Drawing for the job (mm, zero at the part's lowest x, y, z). A direction names the side the tool comes from. Give positions to 0.01 mm unless a question says otherwise; leave off trailing zeros. Write each loop counter-clockwise with the first axis right and the second up, starting at its lowest first coordinate (ties: lowest second). Pieces come first, ordered by that corner, then holes. Notation, with made-up numbers: (-6, 42.25) - (52, 42.25) arc R19 ccw to (52, 49.25) - close; hole circle Ø11 at (83.25, 41.5). An arc over 180 degrees is marked (long way). Use CSV: the item, a comma, the result in double quotes.
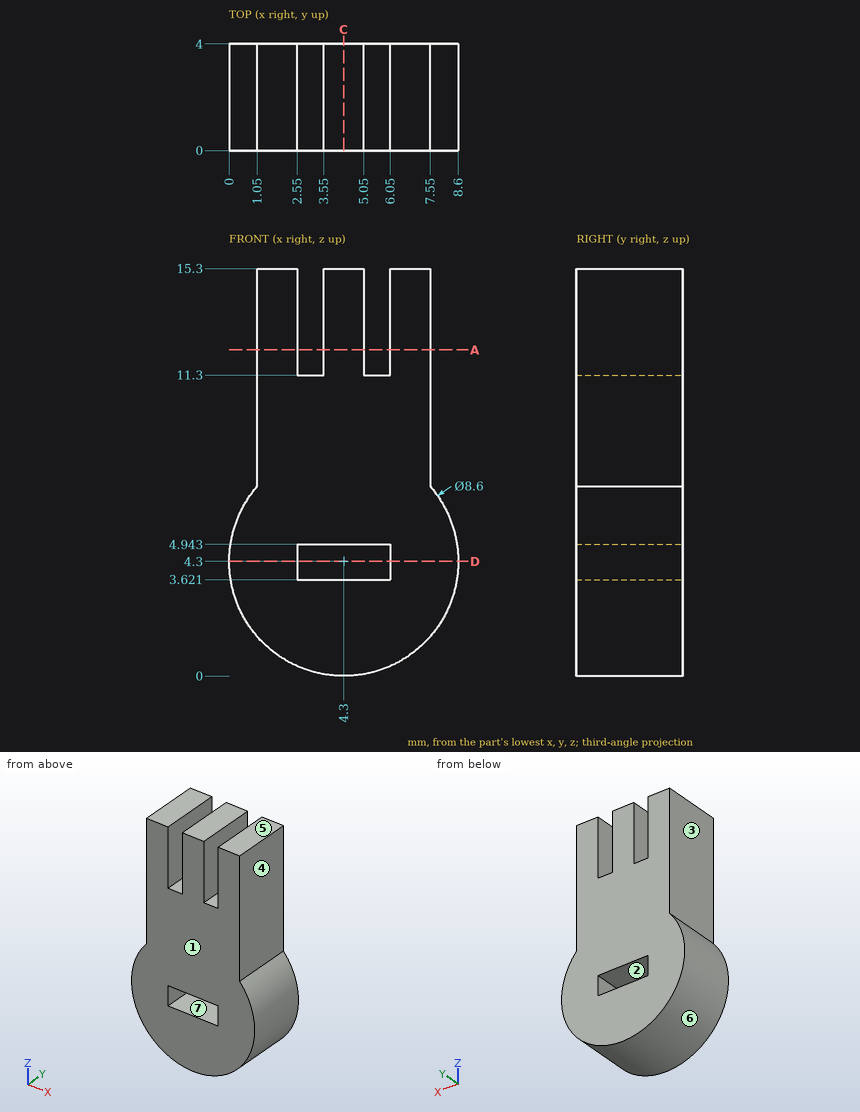
(1) Flat gauge pins, fed straight in: P1, Ø1.5, axis at x = 6, z = 13.5, coming from the -Y side; P2, Ø1.2, axis at y = 1, z = 10.5, coming from the -X side. Where does each tip first touch, or does it go through?
Checked values:
P1,"stops at y = 0"
P2,"stops at x = 1.05"
(2) Saw through at C-C, the plane x = 4.3. List the corners of the cut face in (y, z), then the cut area to 3 significant figures.
Checked values:
outline,"(0, 0) - (4, 0) - (4, 3.62) - (0, 3.62) - close; (0, 4.94) - (4, 4.94) - (4, 15.3) - (0, 15.3) - close"
area,"55.9 mm^2"
(3) Saw through at A-A, the plane z = 12.25. List the corners of the cut face in (x, y).
Checked values:
outline,"(1.05, 0) - (2.55, 0) - (2.55, 4) - (1.05, 4) - close; (3.55, 0) - (5.05, 0) - (5.05, 4) - (3.55, 4) - close; (6.05, 0) - (7.55, 0) - (7.55, 4) - (6.05, 4) - close"
(4) Saw through at D-D, the plane z = 4.3. List the corners of the cut face in (x, y).
Checked values:
outline,"(0, 0) - (2.55, 0) - (2.55, 4) - (0, 4) - close; (6.05, 0) - (8.6, 0) - (8.6, 4) - (6.05, 4) - close"
(5) Pull direction Z, two halves, no side cores. Call the marked faces 4, 5, 6 and 7: released by +Z, released by -Z, zero draft, split by the parting line, or undercut.
Checked values:
face 4,"zero draft"
face 5,"released by +Z"
face 6,"split by the parting line"
face 7,"undercut"
(6) Wall check: probe 1 along X at (y, z) = (1.2, 14.5); probe 2 along X at (y, z) = (0.35, 8.25); probe 3 along Z at (x, y) = (5.5, 3.85). Give the ranges that are in metal, low to high. Write a range as [from, to].
Checked values:
probe 1,"x = [1.05, 2.55], [3.55, 5.05], [6.05, 7.55]"
probe 2,"x = [1.05, 7.55]"
probe 3,"z = [0.17, 3.62], [4.94, 11.3]"
(7) 3-axis set-ups, long thin cutter, end or side, ignore diameter. For the marked faces 1, 2 and 3: which of +Z, -Z, +X, -X, +Y, -Y reach the whole face in a straight line?
Checked values:
face 1,"+Z, -Z, +X, -X, -Y"
face 2,"+Y, -Y"
face 3,"+Z, -X, +Y, -Y"
